The listing builds one solid part. Answer for the finished solid, in the listing's coordinates (mm). Coordinates: 2 decimals unless noted, no trailing zeros. Write each loop counter-clockwise with the first axis right and the second up, starting at its lowest first coordinate (ties: lowest second). Pieces come first, ordered by that corner, then holes. Notation, with made-up numbers: M -22.5,32 L 5.5,32 A7 cw 5.5,42 Z; hole C 48,87.5 d10. An arc over 180 degrees is marked long. Answer as CSV lines item,"result".
```python
from build123d import *

# Parameters (mm, degrees)
F0_R     = 4
F1_DEPTH = 12


with BuildPart() as f1:
    # F0 (on Front) → F1 (new body)
    with BuildSketch(Plane.XZ):
        with BuildLine():
            Line((183.606194, 50), (-180.990682, 50))
            ThreePointArc((-180.990682, 50), (-185.497198, 47.165944), (-184.895026, 41.876525))
            Line((-184.895026, 41.876525), (-152.895026, 1.876525))
            ThreePointArc((-152.895026, 1.876525), (-151.156626, 0.493484), (-148.990682, 0))
            Line((-148.990682, 0), (183.606194, 0))
            ThreePointArc((183.606194, 0), (187.141728, 1.464466), (188.606194, 5))
            Line((188.606194, 5), (188.606194, 45))
            ThreePointArc((188.606194, 45), (187.141728, 48.535534), (183.606194, 50))
        make_face()
        with Locations((-89.263029, 9.591162)):
            Circle(F0_R, mode=Mode.SUBTRACT)
        with BuildLine():
            Line((-133.928709, 46), (-124.089315, 46))
            ThreePointArc((-124.089315, 46), (-121.350702, 45.1833), (-119.506739, 43))
            ThreePointArc((-119.506739, 43), (-117.521867, 39.692195), (-114.759012, 37))
            ThreePointArc((-114.759012, 37), (-111.81474, 33.472136), (-110.759012, 29))
            Line((-110.759012, 29), (-110.759012, 19))
            ThreePointArc((-110.759012, 19), (-115.15241, 8.393398), (-125.759012, 4))
            Line((-125.759012, 4), (-132.259012, 4))
            ThreePointArc((-132.259012, 4), (-142.865614, 8.393398), (-147.259012, 19))
            Line((-147.259012, 19), (-147.259012, 29))
            ThreePointArc((-147.259012, 29), (-146.203284, 33.472136), (-143.259012, 37))
            ThreePointArc((-143.259012, 37), (-140.496156, 39.692195), (-138.511285, 43))
            ThreePointArc((-138.511285, 43), (-136.667322, 45.1833), (-133.928709, 46))
        make_face(mode=Mode.SUBTRACT)
        with BuildLine():
            Line((-42.617198, 46), (-32.777804, 46))
            ThreePointArc((-32.777804, 46), (-30.039191, 45.1833), (-28.195228, 43))
            ThreePointArc((-28.195228, 43), (-26.210357, 39.692195), (-23.447501, 37))
            ThreePointArc((-23.447501, 37), (-20.503229, 33.472136), (-19.447501, 29))
            Line((-19.447501, 29), (-19.447501, 19))
            ThreePointArc((-19.447501, 19), (-23.840899, 8.393398), (-34.447501, 4))
            Line((-34.447501, 4), (-40.947501, 4))
            ThreePointArc((-40.947501, 4), (-51.554103, 8.393398), (-55.947501, 19))
            Line((-55.947501, 19), (-55.947501, 29))
            ThreePointArc((-55.947501, 29), (-54.891773, 33.472136), (-51.947501, 37))
            ThreePointArc((-51.947501, 37), (-49.184646, 39.692195), (-47.199774, 43))
            ThreePointArc((-47.199774, 43), (-45.355811, 45.1833), (-42.617198, 46))
        make_face(mode=Mode.SUBTRACT)
        with Locations((4.899797, 11.972248)):
            Circle(F0_R, mode=Mode.SUBTRACT)
        with Locations((89.348912, 9.877115)):
            Circle(F0_R, mode=Mode.SUBTRACT)
        with Locations((180.782542, 10.067379)):
            Circle(F0_R, mode=Mode.SUBTRACT)
        with BuildLine():
            Line((49.082204, 46), (58.921599, 46))
            ThreePointArc((58.921599, 46), (61.660212, 45.1833), (63.504174, 43))
            ThreePointArc((63.504174, 43), (65.489046, 39.692195), (68.251902, 37))
            ThreePointArc((68.251902, 37), (71.196173, 33.472136), (72.251902, 29))
            Line((72.251902, 29), (72.251902, 19))
            ThreePointArc((72.251902, 19), (67.858503, 8.393398), (57.251902, 4))
            Line((57.251902, 4), (50.751902, 4))
            ThreePointArc((50.751902, 4), (40.1453, 8.393398), (35.751902, 19))
            Line((35.751902, 19), (35.751902, 29))
            ThreePointArc((35.751902, 29), (36.80763, 33.472136), (39.751902, 37))
            ThreePointArc((39.751902, 37), (42.514757, 39.692195), (44.499629, 43))
            ThreePointArc((44.499629, 43), (46.343592, 45.1833), (49.082204, 46))
        make_face(mode=Mode.SUBTRACT)
        with Locations((-176.895979, 42)):
            Circle(F0_R, mode=Mode.SUBTRACT)
        with Locations((-76.374538, 43)):
            Circle(F0_R, mode=Mode.SUBTRACT)
        with BuildLine():
            Line((140.436497, 46), (150.275891, 46))
            ThreePointArc((150.275891, 46), (153.014504, 45.1833), (154.858467, 43))
            ThreePointArc((154.858467, 43), (156.843338, 39.692195), (159.606194, 37))
            ThreePointArc((159.606194, 37), (162.550466, 33.472136), (163.606194, 29))
            Line((163.606194, 29), (163.606194, 19))
            ThreePointArc((163.606194, 19), (159.212796, 8.393398), (148.606194, 4))
            Line((148.606194, 4), (142.106194, 4))
            ThreePointArc((142.106194, 4), (131.499592, 8.393398), (127.106194, 19))
            Line((127.106194, 19), (127.106194, 29))
            ThreePointArc((127.106194, 29), (128.161922, 33.472136), (131.106194, 37))
            ThreePointArc((131.106194, 37), (133.869049, 39.692195), (135.853921, 43))
            ThreePointArc((135.853921, 43), (137.697884, 45.1833), (140.436497, 46))
        make_face(mode=Mode.SUBTRACT)
        with Locations((18.551346, 43)):
            Circle(F0_R, mode=Mode.SUBTRACT)
        with Locations((104.270376, 43)):
            Circle(F0_R, mode=Mode.SUBTRACT)
    extrude(amount=F1_DEPTH)


solid = f1.part
```
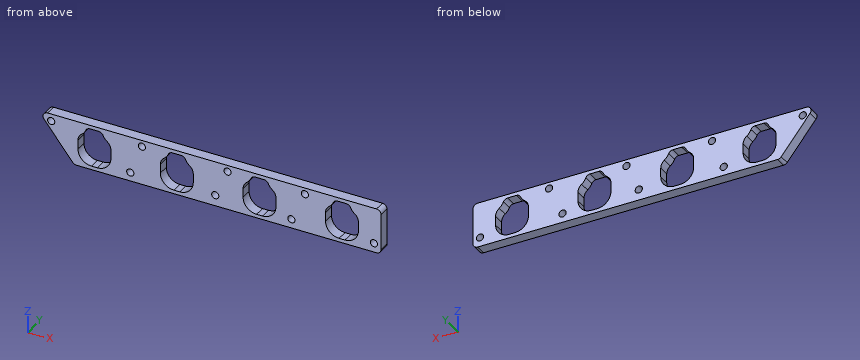
Q1. Flat-ended cylindrical pins translate along their axes: pin 1 Ø5 at (y, z) = (-7.5, 6.5) entering from -X; pin 2 Ø3 at (y, z) = (-9, 22) entering from -X; pin 3 Ø5 at (y, z) = (-5, 22) entering from -X. Find the tip coordinate at first contact, or state that the pin passes through.
Output:
pin 1,"x = -158.59"
pin 2,"x = -170.19"
pin 3,"x = -170.99"
Q2. Find section A-A (x = 89). Give the vertices of the cut face in (y, z), and give its area (3 significant figures).
Output:
outline,"M -12,0 L 0,0 L 0,5.89 L -12,5.89 Z; M -12,13.86 L 0,13.86 L 0,50 L -12,50 Z"
area,"504 mm2"
Q3. Straight lines are drawn through the part: line 1 (X direction, y = -7.25, z = 32.5) (1 decimal); line 2 (X direction, y = -10.5, z = 23); line 3 (Z direction, x = 57, y = -4). For each, find the intervals that lie inside material, in ascending order.
Output:
line 1,"-177.4 to -146.6, -111.4 to -55.3, -20.1 to 36.4, 71.6 to 127.7, 163 to 188.6"
line 2,"-169.79 to -147.26, -110.76 to -55.95, -19.45 to 35.75, 72.25 to 127.11, 163.61 to 188.61"
line 3,"0 to 4, 46 to 50"
Q4. Find section B-B (y = -7). Count the separate pieces of the cut face and the enclosed holes in it, and give its area (3 significant figures).
Output:
separate pieces,"1"
enclosed holes,"12"
area,"12,500 mm2"
